Could you check a few things on this drawing? It's one solid part, dimensions in mm from its lowest x, y, z. Round coordinates to 2 decimals unless told otherwise and drop trailing zeros. Write each loop counter-clockwise with the first axis right and the second up, starting at its lowest first coordinate (ties: lowest second). Pieces come first, ordered by that corner, then holes. Notation, with made-up numbers: (73, 74.5) -> (86, 74.5) arc R22 cw to (86, 94.5) -> close; hole circle Ø2 at (-3, 1.25). An arc over 180 degrees is marked (long way). Answer as CSV lines item,"result".
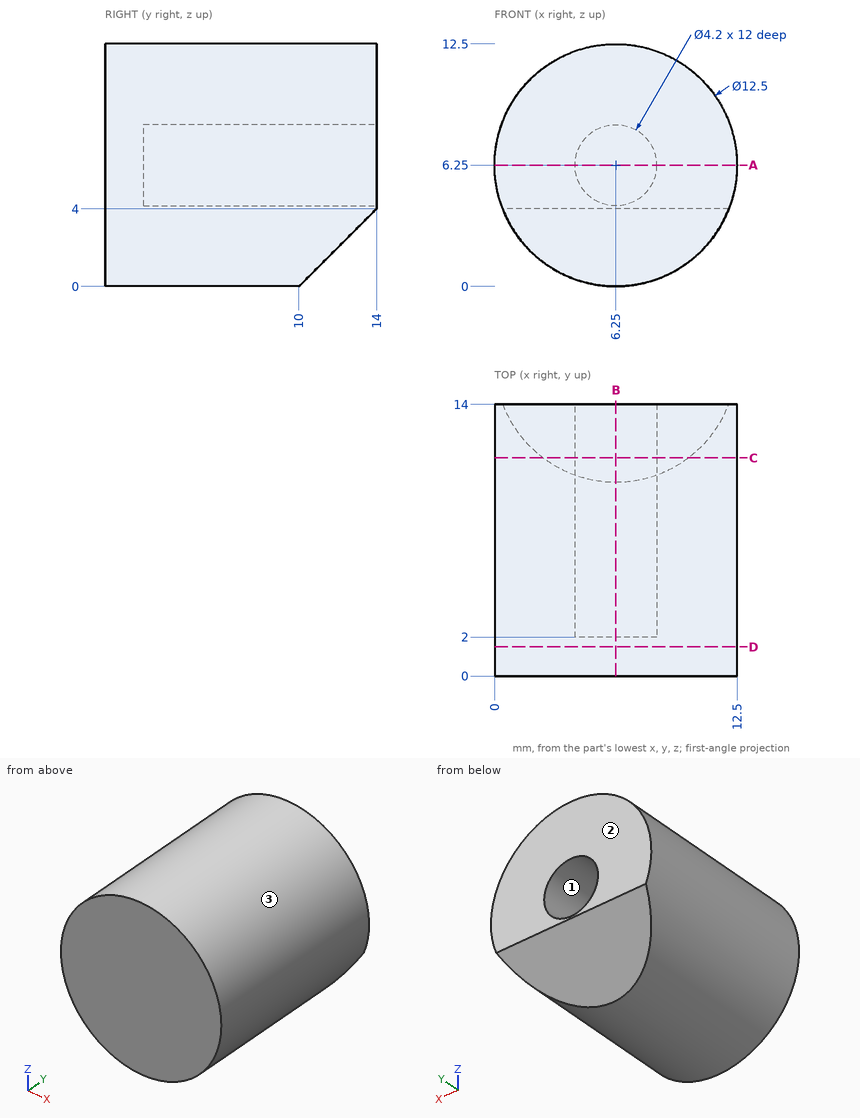
1. Suppose I cut it at D-D on y = 1.5. Please give me the cut outline in (x, z), and give its area (3 significant figures).
Numbers:
outline,"circle Ø12.5 at (6.25, 6.25)"
area,"123 mm^2"
2. Suppose I cut it at A-A on z = 6.25. Please give me the cut outline in (x, y).
Numbers:
outline,"(0, 0) -> (12.5, 0) -> (12.5, 14) -> (8.35, 14) -> (8.35, 2) -> (4.15, 2) -> (4.15, 14) -> (0, 14) -> close"
3. For pin 1 Ø1 at (x, y) = (7.5, 8.5) entering from -Z; pin 2 Ø1 at (y, z) = (12.5, 3) entering from +X, each with a flat end and sliding along its axis, tell me the tip position at first contact or that it passes through.
Numbers:
pin 1,"stops at z = 0.05"
pin 2,"stops at x = 11.86"
4. If I drill on line 1 (Z direction, x = 6.25, y = 9.5); line 2 (Z direction, x = 7, y = 10.5), over which ranges is the centre line in solid material (lowest first)?
Numbers:
line 1,"z = 0 to 4.15, 8.35 to 12.5"
line 2,"z = 0.5 to 4.29, 8.21 to 12.45"
5. If we mould it in two halves opening along X, with no side actions, what happens to the marked faces 1, 2 and 3? For each: released by +X, released by -X, zero draft, split by the parting line, or undercut.
Numbers:
face 1,"undercut"
face 2,"zero draft"
face 3,"split by the parting line"
6. Suppose I cut it at C-C on y = 11.25. Please give me the cut outline in (x, z).
Numbers:
outline,"(2.5, 1.25) -> (10, 1.25) arc R6.25 ccw (long way) to start; hole circle Ø4.2 at (6.25, 6.25)"
7. Suppose I cut it at B-B on x = 6.25. Please give me the cut outline in (y, z).
Numbers:
outline,"(0, 0) -> (10, 0) -> (14, 4) -> (14, 4.15) -> (2, 4.15) -> (2, 8.35) -> (14, 8.35) -> (14, 12.5) -> (0, 12.5) -> close"
